Input: part model. Units: mm. Frame: model coordinates. Face numbers are marked on the shaded views. A direction names the side the tool comes from. Round coordinates to 2 decimals unless told otherwise and drop trailing zeros. Loops run counter-clockwise (first coordinate to the right, second up) from the corner with the lowest first, then second, coordinate; pieces in that order, holes last.
1) Access query for the marked faces 5, 6 and 7. Directions: +Z, -Z, +X, -X, +Y, -Y. A direction counts if a zero-diameter tool reaches every point of the face in a straight line with its end or side. Return the directions, or none.
2) Section D-D, the plane z = -15. Return loops of the section in (x, y).
3) Ray query, line 1 along X through (y, z) = (3.9, -30); line 2 along X through (y, z) = (31, -15); line 3 along Y through (x, z) = (6, -27). Return the intervals inside material, ascending.
4) Section A-A, the plane y = 14. Return loops of the section in (x, z).
5) Draft query along Z for the marked faces 1, 2, 3 and 4. Return one class per face: pulls with the +Z half, pulls with the -Z half, needs draft (parallel to the pull), parting line crosses it, or undercut.
6) Section B-B, the plane z = -23. Return loops of the section in (x, y).
7) Section C-C, the plane x = 4. Return loops of the section in (y, z).
8) First-contact query: pin 1 (3 mm diameter, centred on x = 13, y = 20.5, fed in from +Z); pin 2 (4.5 mm diameter, centred on x = 14.5, y = 20.5, fed in from -Z); pin 3 (2 mm diameter, centred on x = 27.5, z = -5, fed in from +Y). Flat tips, straight axial feed; report the tip coordinate or a pass-through.
from build123d import *

# Parameters (mm, degrees)
SKETCH1_W           = 35
SKETCH1_H           = 40
SKETCH1_R           = 1.25
BOSS_EXTRUDE1_DEPTH = 5
FILLET1_R           = 8
FILLET2_R           = 8
SKETCH2_W           = 8
SKETCH2_H           = 10
BOSS_EXTRUDE2_DEPTH = 30
RIB1_REACH          = 62.622
SKETCH4_WALL_W      = 154.866333132
SKETCH4_WALL_H      = 4
BOSS_EXTRUDE3_REACH = 59.879
SKETCH5_W           = 8
SKETCH5_H           = 7
CUT_EXTRUDE1_REACH  = 65.64
SKETCH6_R           = 1.4
FILLET7_R           = 1
FILLET8_R           = 2


with BuildPart() as part:
    # Sketch1 → Boss-Extrude1 (new body)
    with BuildSketch(Plane(origin=(0, 0, 0), x_dir=(1, 0, 0), z_dir=(0, 1, 0))):
        with Locations((17.5, 20)):
            Rectangle(SKETCH1_W, SKETCH1_H)
        with Locations(Location((26.160254038, 30, 0), (0, 0, 270))):
            Circle(SKETCH1_R, mode=Mode.SUBTRACT)
        with Locations(Location((8.839745962, 20, 0), (0, 0, 270))):
            Circle(SKETCH1_R, mode=Mode.SUBTRACT)
        with Locations(Location((26.160254038, 10, 0), (0, 0, 270))):
            Circle(SKETCH1_R, mode=Mode.SUBTRACT)
    extrude(amount=BOSS_EXTRUDE1_DEPTH)

    # Fillet1
    fillet1_edges = [part.edges().sort_by_distance(p)[0] for p in [
        (35, 2.5, 0),
    ]]
    fillet(fillet1_edges, radius=FILLET1_R)

    # Fillet2
    fillet2_edges = [part.edges().sort_by_distance(p)[0] for p in [
        (35, 2.5, -40),
    ]]
    fillet(fillet2_edges, radius=FILLET2_R)

    # Sketch2 → Boss-Extrude2 (add)
    with BuildSketch(Plane(origin=(0, 5, 0), x_dir=(1, 0, 0), z_dir=(0, 1, 0))):
        with Locations((4, 5)):
            Rectangle(SKETCH2_W, SKETCH2_H)
        with Locations((4, 35)):
            Rectangle(SKETCH2_W, SKETCH2_H)
    extrude(amount=BOSS_EXTRUDE2_DEPTH)

    # Sketch4 wall → Rib1 (add, up to next)
    with BuildSketch(Plane(origin=(13, 20, -5), x_dir=(0.316227766017, -0.948683298051, 0), z_dir=(0.948683298051, 0.316227766017, 0)), mode=Mode.PRIVATE) as rib1_sk1:
        Rectangle(SKETCH4_WALL_W, SKETCH4_WALL_H)
    rib1_tool1 = extrude(rib1_sk1.sketch, amount=-RIB1_REACH, mode=Mode.PRIVATE) - part.part
    rib1 = rib1_tool1.solids().sort_by_distance((13, 20, -5))[0]
    add(rib1)

    # Mirror2: Rib1 across plane
    add(rib1.mirror(Plane(origin=(0, 0, -20), x_dir=(1, 0, 0), z_dir=(0, 0, -1))))

    # Sketch5 → Boss-Extrude3 (add, up to next)
    with BuildSketch(Plane.XY.offset(-30), mode=Mode.PRIVATE) as boss_extrude3_sk1:
        with Locations((4, 31.5)):
            Rectangle(SKETCH5_W, SKETCH5_H)
    boss_extrude3_tool1 = extrude(boss_extrude3_sk1.sketch, amount=BOSS_EXTRUDE3_REACH, mode=Mode.PRIVATE) - part.part
    add(boss_extrude3_tool1.solids().sort_by_distance((4, 31.5, -30))[0])

    # Sketch6 → Cut-Extrude1 (cut, up to next)
    with BuildSketch(Plane(origin=(0, 35, 0), x_dir=(1, 0, 0), z_dir=(0, 1, 0)), mode=Mode.PRIVATE) as cut_extrude1_sk1:
        with Locations(Location((4, 15, 0), (0, 0, 270))):
            Circle(SKETCH6_R)
    cut_extrude1_tool1 = extrude(cut_extrude1_sk1.sketch, amount=-CUT_EXTRUDE1_REACH, mode=Mode.PRIVATE) & part.part
    # Sketch6 → Cut-Extrude1 (cut, up to next)
    with BuildSketch(Plane(origin=(0, 35, 0), x_dir=(1, 0, 0), z_dir=(0, 1, 0)), mode=Mode.PRIVATE) as cut_extrude1_sk2:
        with Locations(Location((4, 25, 0), (0, 0, 270))):
            Circle(SKETCH6_R)
    cut_extrude1_tool2 = extrude(cut_extrude1_sk2.sketch, amount=-CUT_EXTRUDE1_REACH, mode=Mode.PRIVATE) & part.part
    add(cut_extrude1_tool1.solids().sort_by_distance((4, 35, -15))[0], mode=Mode.SUBTRACT)
    add(cut_extrude1_tool2.solids().sort_by_distance((4, 35, -25))[0], mode=Mode.SUBTRACT)

    # Fillet7
    fillet7_edges = [part.edges().sort_by_distance(p)[0] for p in [
        (8, 20, 0),
        (32.656854249, 5, -37.656854249),
        (17.5, 5, -40),
        (8, 20, -37),
        (13, 5, -37),
        (18, 5, -35),
        (13, 5, -33),
        (8, 5, -31.5),
        (4, 5, -30),
        (4, 5, -10),
        (8, 5, -8.5),
        (35, 5, -20),
        (32.656854249, 5, -2.343145751),
        (8, 20, -3),
        (8, 20, -7),
        (13, 5, -7),
        (18, 5, -5),
        (13, 5, -3),
        (17.5, 5, 0),
        (8, 5, -1.5),
    ]]
    fillet(fillet7_edges, radius=FILLET7_R)

    # Fillet8
    fillet8_edges = [part.edges().sort_by_distance(p)[0] for p in [
        (4, 28, -10),
        (4, 28, -30),
    ]]
    fillet(fillet8_edges, radius=FILLET8_R)


solid = part.part
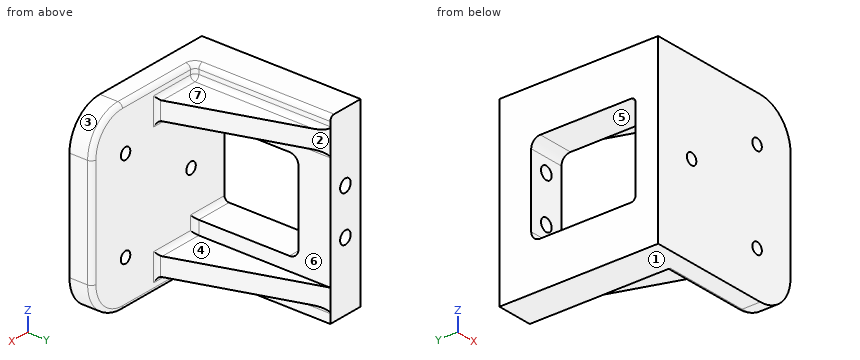
Final values:
1. face 5: +X, -X
1. face 6: +X, +Y
1. face 7: +Z, +X, +Y
2. outline: (0, 0) - (35, 0) - (35, 4) arc R1 ccw to (34, 5) - (0, 5) - close; (0, 28) - (2.6, 28) - (2.6, 35) - (0, 35) - close; (5.4, 28) - (8, 28) - (8, 35) - (5.4, 35) - close
3. line 1: x = 0 to 24.91, 27.41 to 35
3. line 2: x = 0 to 2.6, 5.4 to 8
3. line 3: y = 0 to 5, 28 to 35
4. outline: (0, -40) - (8, -40) - (8, -38) arc R1 cw to (9, -37) - (15, -37) - (15, -33) - (8, -33) - (8, -30) - (0, -30) - close; (0, -10) - (8, -10) - (8, -8) arc R1 cw to (9, -7) - (15, -7) - (15, -3) - (9, -3) arc R1 cw to (8, -2) - (8, -1) arc R1 ccw to (7, 0) - (0, 0) - close
5. face 1: pulls with the -Z half
5. face 2: needs draft
5. face 3: pulls with the +Z half
5. face 4: undercut
6. outline: (0, 0) - (35, 0) - (35, 4) arc R1 ccw to (34, 5) - (0, 5) - close; (0, 28) - (8, 28) - (8, 35) - (0, 35) - close
7. outline: (0, -40) - (35, -40) - (35, -26.4) - (28, -26.4) - (28, -28) arc R2 cw to (26, -30) - (6, -30) arc R1 cw to (5, -29) - (5, -11) arc R1 cw to (6, -10) - (26, -10) arc R2 cw to (28, -12) - (28, -13.6) - (35, -13.6) - (35, 0) - (0, 0) - close; (28, -23.6) - (35, -23.6) - (35, -16.4) - (28, -16.4) - close
8. pin 1: stops at z = -3
8. pin 2: stops at z = -37
8. pin 3: stops at y = 5
